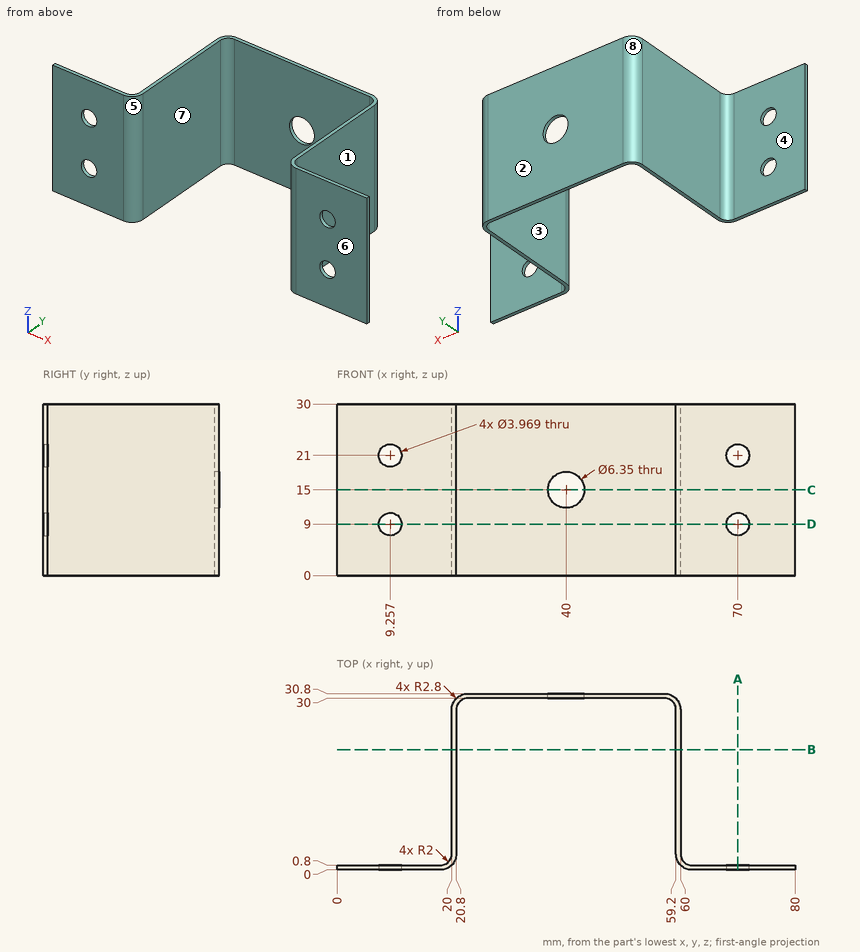
Drawing for the job (mm, zero at the part's lowest x, y, z). A direction names the side the tool comes from. Round coordinates to 2 decimals unless told otherwise and drop trailing zeros. Write each loop counter-clockwise with the first axis right and the second up, starting at its lowest first coordinate (ties: lowest second). Pieces come first, ordered by that corner, then holes. Notation, with made-up numbers: (1.5, 35.5) - (45.5, 35.5) arc R25 cw to (45.5, 69.5) - close; hole circle Ø9 at (20.5, -36.75). An arc over 180 degrees is marked (long way). Return JSON: item names as keys, results as strings. Group by question number.
Item 1: Mould opens along X. For the marked faces 5, 6, 7 and 8 say: +X half, -X half, draft (parallel to the pull), parting line (faces both ways), or undercut.
Item 2: Band-saw the part on B-B on y = 21. List the corners of the cut face in (x, z).
Item 3: 3-axis set-ups, long thin cutter, end or side, ignore diameter. For the marked faces 1, 2, 3 and 4: which of +Z, -Z, +X, -X, +Y, -Y reach the whole face in a straight line?
Item 4: Flat gauge pins, fed straight in: pin 1 Ø8 at (x, z) = (51.5, 15) entering from -Y; pin 2 Ø7.5 at (y, z) = (17.5, 10.5) entering from -X; pin 3 Ø10 at (x, z) = (55.5, 8.5) entering from -Y (1 decimal). Where does each tip first touch, or does it go through?
Item 5: Band-saw the part on C-C on z = 15. List the corners of the cut face in (x, y) (1 decimal).
Item 6: Probe probe 1 along Z at (x, y) = (70, 0.35); probe 2 along X at (y, z) = (14.5, 13.75); probe 3 along Y at (x, z) = (15, 8.75). List the from-to ranges inside material, lowest first.
Item 7: Band-saw the part on A-A on x = 70. List the corners of the cut face in (y, z).
Item 8: Band-saw the part on D-D on z = 9. List the corners of the cut face in (x, y), plus the area to 3 significant figures.
Resolved:
{
 "1": {"face 5": "undercut", "face 6": "draft", "face 7": "undercut", "face 8": "-X half"},
 "2": {"outline": "(20, 0) - (20.8, 0) - (20.8, 30) - (20, 30) - close; (59.2, 0) - (60, 0) - (60, 30) - (59.2, 30) - close"},
 "3": {"face 1": "+Z, -Z, +X, +Y", "face 2": "+Z, -Z, +X, -X, +Y", "face 3": "+Z, -Z, -Y", "face 4": "+Z, -Z, -X, +Y"},
 "4": {"pin 1": "stops at y = 30", "pin 2": "stops at x = 20", "pin 3": "stops at y = 0.4"},
 "5": {"outline": "(0, 0) - (18, 0) arc R2.8 ccw to (20.8, 2.8) - (20.8, 28) arc R2 cw to (22.8, 30) - (36.8, 30) - (36.8, 30.8) - (22.8, 30.8) arc R2.8 ccw to (20, 28) - (20, 2.8) arc R2 cw to (18, 0.8) - (0, 0.8) - close; (43.2, 30) - (57.2, 30) arc R2 cw to (59.2, 28) - (59.2, 2.8) arc R2.8 ccw to (62, 0) - (80, 0) - (80, 0.8) - (62, 0.8) arc R2 cw to (60, 2.8) - (60, 28) arc R2.8 ccw to (57.2, 30.8) - (43.2, 30.8) - close"},
 "6": {"probe 1": "z = 0 to 7.02, 10.98 to 19.02, 22.98 to 30", "probe 2": "x = 20 to 20.8, 59.2 to 60", "probe 3": "y = 0 to 0.8"},
 "7": {"outline": "(0, 0) - (0.8, 0) - (0.8, 7.02) - (0, 7.02) - close; (0, 10.98) - (0.8, 10.98) - (0.8, 19.02) - (0, 19.02) - close; (0, 22.98) - (0.8, 22.98) - (0.8, 30) - (0, 30) - close"},
 "8": {"outline": "(0, 0) - (7.27, 0) - (7.27, 0.8) - (0, 0.8) - close; (11.24, 0) - (18, 0) arc R2.8 ccw to (20.8, 2.8) - (20.8, 28) arc R2 cw to (22.8, 30) - (57.2, 30) arc R2 cw to (59.2, 28) - (59.2, 2.8) arc R2.8 ccw to (62, 0) - (68.02, 0) - (68.02, 0.8) - (62, 0.8) arc R2 cw to (60, 2.8) - (60, 28) arc R2.8 ccw to (57.2, 30.8) - (22.8, 30.8) arc R2.8 ccw to (20, 28) - (20, 2.8) arc R2 cw to (18, 0.8) - (11.24, 0.8) - close; (71.98, 0) - (80, 0) - (80, 0.8) - (71.98, 0.8) - close", "area": "102 mm²"}
}
